```python
from build123d import *

# Parameters (mm, degrees)
BOSS_EXTRUDE1_DEPTH       = 51
BOSS_EXTRUDE2_DEPTH       = 51
SKETCH1_4_R               = 4.5
BOSS_EXTRUDE3_DEPTH       = 9
CUT_EXTRUDE1_REACH        = 98.057
SKETCH2_R                 = 4.5
BOSS_EXTRUDE4_START       = -42
SKETCH3_R                 = 8
BOSS_EXTRUDE4_DEPTH       = 42
F_6_0MM_DOWEL_HOLE1_D     = 6
F_6_0MM_DOWEL_HOLE1_DEPTH = 13


with BuildPart() as part:
    # Sketch1 → Boss-Extrude1 (new body)
    with BuildSketch(Plane.XY):
        with BuildLine():
            ThreePointArc((40, 0), (39.453405592, 6.590052141), (37.828560639, 13))
            ThreePointArc((37.828560639, 13), (0, 40), (-37.828560639, 13))
            ThreePointArc((-37.828560639, 13), (-39.453405592, 6.590052141), (-40, 0))
            Line((-40, 0), (-26.965, 0))
            ThreePointArc((-26.965, 0), (0, 26.965), (26.965, 0))
            Line((26.965, 0), (40, 0))
        make_face()
    extrude(amount=BOSS_EXTRUDE1_DEPTH)

    # Sketch1<3> → Boss-Extrude2 (add)
    with BuildSketch(Plane.XY):
        with BuildLine():
            Line((63.686733312, 13), (37.828560639, 13))
            ThreePointArc((37.828560639, 13), (39.453405592, 6.590052141), (40, 0))
            Line((40, 0), (65, 0))
            Line((65, 0), (65, 13))
            Line((65, 13), (63.686733312, 13))
        make_face()
        with BuildLine():
            ThreePointArc((-40, 0), (-39.453405592, 6.590052141), (-37.828560639, 13))
            Line((-37.828560639, 13), (-63.686733312, 13))
            Line((-63.686733312, 13), (-65, 13))
            Line((-65, 13), (-65, 0))
            Line((-65, 0), (-40, 0))
        make_face()
    extrude(amount=BOSS_EXTRUDE2_DEPTH)

    # Sketch1<4> → Boss-Extrude3 (add)
    with BuildSketch(Plane.XY):
        with BuildLine():
            ThreePointArc((-37.828560639, 13), (0, 40), (37.828560639, 13))
            Line((37.828560639, 13), (63.686733312, 13))
            ThreePointArc((63.686733312, 13), (48.281028578, 43.519447141), (19.519221296, 62))
            Line((19.519221296, 62), (-19.519221296, 62))
            ThreePointArc((-19.519221296, 62), (-48.281028578, 43.519447141), (-63.686733312, 13))
            Line((-63.686733312, 13), (-37.828560639, 13))
        make_face()
        with Locations((-41, 32)):
            Circle(SKETCH1_4_R, mode=Mode.SUBTRACT)
        with Locations((41, 32)):
            Circle(SKETCH1_4_R, mode=Mode.SUBTRACT)
    extrude(amount=BOSS_EXTRUDE3_DEPTH)

    # Sketch2 → Cut-Extrude1 (cut, up to next)
    with BuildSketch(Plane(origin=(0, 13, 0), x_dir=(1, 0, 0), z_dir=(0, 1, 0)), mode=Mode.PRIVATE) as cut_extrude1_sk1:
        with Locations(Location((52, -21, 0), (0, 0, 180))):
            Circle(SKETCH2_R)
    cut_extrude1_tool1 = extrude(cut_extrude1_sk1.sketch, amount=-CUT_EXTRUDE1_REACH, mode=Mode.PRIVATE) & part.part
    # Sketch2 → Cut-Extrude1 (cut, up to next)
    with BuildSketch(Plane(origin=(0, 13, 0), x_dir=(1, 0, 0), z_dir=(0, 1, 0)), mode=Mode.PRIVATE) as cut_extrude1_sk2:
        with Locations(Location((-52, -21, 0), (0, 0, 180))):
            Circle(SKETCH2_R)
    cut_extrude1_tool2 = extrude(cut_extrude1_sk2.sketch, amount=-CUT_EXTRUDE1_REACH, mode=Mode.PRIVATE) & part.part
    # Sketch2 → Cut-Extrude1 (cut, up to next)
    with BuildSketch(Plane(origin=(0, 13, 0), x_dir=(1, 0, 0), z_dir=(0, 1, 0)), mode=Mode.PRIVATE) as cut_extrude1_sk3:
        with BuildLine():
            Line((65, -51), (65, -21))
            ThreePointArc((65, -21), (63.859756378, -26.324112946), (60.639049437, -30.714258841))
            Line((60.639049437, -30.714258841), (37.828560639, -51))
            Line((37.828560639, -51), (65, -51))
        make_face()
    cut_extrude1_tool3 = extrude(cut_extrude1_sk3.sketch, amount=-CUT_EXTRUDE1_REACH, mode=Mode.PRIVATE) & part.part
    # Sketch2 → Cut-Extrude1 (cut, up to next)
    with BuildSketch(Plane(origin=(0, 13, 0), x_dir=(1, 0, 0), z_dir=(0, 1, 0)), mode=Mode.PRIVATE) as cut_extrude1_sk4:
        with BuildLine():
            Line((-65, -51), (-37.828560639, -51))
            Line((-37.828560639, -51), (-60.639049437, -30.714258841))
            ThreePointArc((-60.639049437, -30.714258841), (-63.859756378, -26.324112946), (-65, -21))
            Line((-65, -21), (-65, -51))
        make_face()
    cut_extrude1_tool4 = extrude(cut_extrude1_sk4.sketch, amount=-CUT_EXTRUDE1_REACH, mode=Mode.PRIVATE) & part.part
    add(cut_extrude1_tool1.solids().sort_by_distance((52, 13, 21))[0], mode=Mode.SUBTRACT)
    add(cut_extrude1_tool2.solids().sort_by_distance((-52, 13, 21))[0], mode=Mode.SUBTRACT)
    add(cut_extrude1_tool3.solids().sort_by_distance((56.054542, 13, 42.719243))[0], mode=Mode.SUBTRACT)
    add(cut_extrude1_tool4.solids().sort_by_distance((-56.054542, 13, 42.719243))[0], mode=Mode.SUBTRACT)

    # Sketch3 → Boss-Extrude4 (add)
    with BuildSketch(Plane.XY.offset(51).offset(BOSS_EXTRUDE4_START)):
        with Locations((-36, 14)):
            Circle(SKETCH3_R)
    extrude(amount=BOSS_EXTRUDE4_DEPTH)

    # Ø6.0mm Dowel Hole1
    with Locations(Plane.XY.offset(51)):
        with Locations((-36, 14)):
            Hole(F_6_0MM_DOWEL_HOLE1_D / 2, depth=F_6_0MM_DOWEL_HOLE1_DEPTH)


solid = part.part
```
Geometry check sheet. Reference: the model listing, model coordinates, mm. A direction names the side the tool comes from. Coordinates: 2 decimals unless noted, no trailing zeros. Loops run counter-clockwise (first coordinate to the right, second up) from the corner with the lowest first, then second, coordinate; pieces in that order, holes last.
Item 1: Sectioned sample at A-A, the plane z = 3. Record the boundary of the cut face in (x, y) (3 decimals), then the cut area to 3 significant figures.
Item 2: Release check for a two-part mould opening along Z. For faces 4 (the face through (-49.074, 6.591, 40.999)), 5 (the face through (-54.419, 6.591, 24.794)), 6 (the face through (-33, 14, 44)) record: released by +Z, released by -Z, zero draft, split by the parting line, or undercut.
Item 3: Sectioned sample at C-C, the plane y = 25. Record the boundary of the cut face in (x, z) (3 decimals).
Item 4: Sectioned sample at D-D, the plane y = 32. Record the boundary of the cut face in (x, z), then the cut area to 3 significant figures.
Item 5: Access from +Z, -Z, +X, -X, +Y, -Y to the whole of each face (thin tool, end or side, straight path). Record for faces 1 (the face through (-1, 43, 9)), 2 (the face through (-0.59, 26.96, 25.14)), 3 (the face through (49, 13, 25)).
Item 6: Go/stop test with flat-tipped pins: pin 1 Ø11.5 at (x, z) = (52, 21) entering from +Y; pin 2 Ø2 at (x, z) = (12, 31.5) entering from -Y; pin 3 Ø1.8 at (x, y) = (-36, 14.5) entering from +Z. Record where each tip stops, or that it passes through.
Item 7: Thickness scan on line 1 (Y direction, x = -47, z = 42); line 2 (Z direction, x = 31, y = 47); line 3 (X direction, y = 24, z = 23). Record the ranges inside material, lowest first.
Item 8: Sectioned sample at B-B, the plane x = 41. Record the boundary of the cut face in (y, z).
Check result:
1. outline: (-65, 0) - (-26.965, 0) arc R26.965 cw to (26.965, 0) - (65, 0) - (65, 13) - (63.687, 13) arc R65 ccw to (19.519, 62) - (-19.519, 62) arc R65 ccw to (-63.687, 13) - (-65, 13) - close; hole circle Ø9 at (-41, 32); hole circle Ø9 at (41, 32)
1. area: 5,300 mm2
2. face 4: released by +Z
2. face 5: undercut
2. face 6: zero draft
3. outline: (-60, 0) - (-10.105, 0) - (-10.105, 51) - (-31.225, 51) - (-31.225, 9) - (-60, 9) - close; (10.105, 0) - (60, 0) - (60, 9) - (31.225, 9) - (31.225, 51) - (10.105, 51) - close
4. outline: (-56.58, 0) - (-45.5, 0) - (-45.5, 9) - (-56.58, 9) - close; (-36.5, 0) - (36.5, 0) - (36.5, 9) - (24, 9) - (24, 51) - (-24, 51) - (-24, 9) - (-36.5, 9) - close; (45.5, 0) - (56.58, 0) - (56.58, 9) - (45.5, 9) - close
4. area: 2,870 mm2
5. face 1: +Z, +Y
5. face 2: +Z, -Z, -Y
5. face 3: +Z, +X, +Y
6. pin 1: stops at y = 13
6. pin 2: stops at y = 23.62
6. pin 3: stops at z = 38
7. line 1: y = 0 to 13
7. line 2: z = 0 to 9
7. line 3: x = -32 to -12.29, 12.29 to 32
8. outline: (0, 0) - (27.5, 0) - (27.5, 9) - (13, 9) - (13, 48.18) - (0, 48.18) - close; (36.5, 0) - (50.44, 0) - (50.44, 9) - (36.5, 9) - close
